Geometry: see drawing. Coordinates: mm, zero at the bounding-box minimum. Give positions to 0.01 mm unless a question says otherwise; leave off trailing zeros. Order: outer loops, then holes, each group sorted by start corner. A loop starts at its lowest first (then second) coordinate and runs counter-clockwise, first axis right, second up. Notation, with made-up numbers: M 42.5,-2 L 61.5,-2 A24 ccw 61.5,34 Z; hole C 73,39 d10. An arc over 180 degrees is marked long. Return JSON: item names as keys, results as strings.
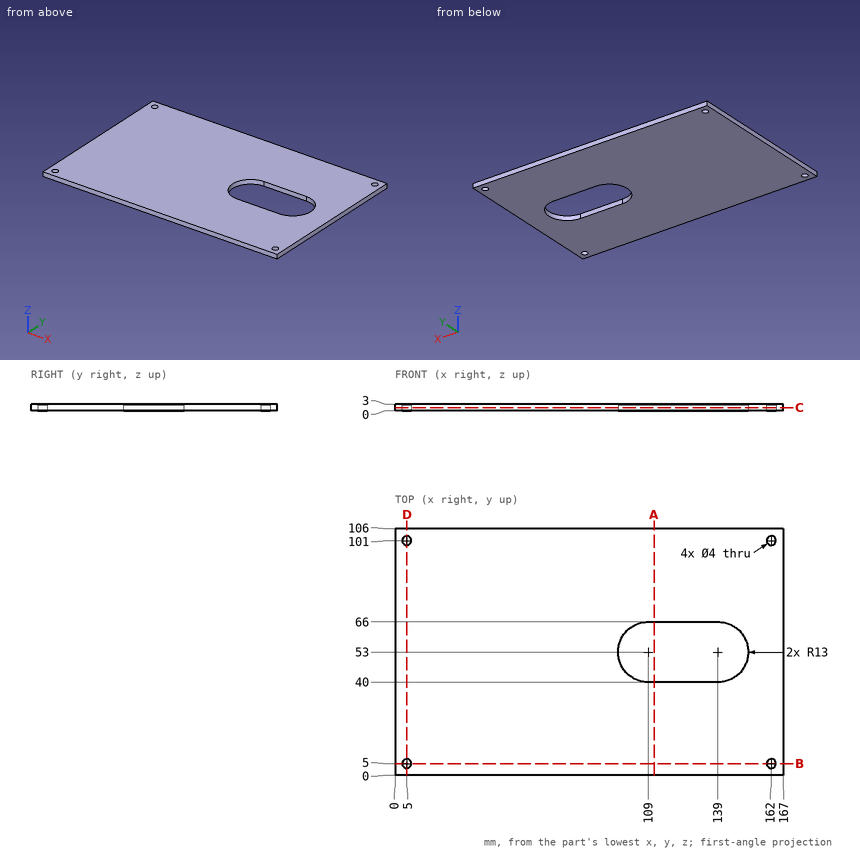
1. Section query D-D (x = 5). Return loops of the section in (y, z), then the cut area to 3 significant figures.
Evaluation:
{"outline": "M 0,0 L 3,0 L 3,3 L 0,3 Z; M 7,0 L 99,0 L 99,3 L 7,3 Z; M 103,0 L 106,0 L 106,3 L 103,3 Z", "area": "294 mm^2"}
2. Ray query, probe 1 along Y at (x, z) = (162, 1.75); probe 2 along X at (y, z) = (101, 1.2); probe 3 along Y at (x, z) = (119, 2.45). Return the intervals inside material, ascending.
Evaluation:
{"probe 1": "y = 0 to 3, 7 to 99, 103 to 106", "probe 2": "x = 0 to 3, 7 to 160, 164 to 167", "probe 3": "y = 0 to 40, 66 to 106"}
3. Section query C-C (z = 1.4). Return loops of the section in (x, y).
Evaluation:
{"outline": "M 0,0 L 167,0 L 167,106 L 0,106 Z; hole C 5,5 d4; hole C 5,101 d4; hole M 109,40 L 139,40 A13 ccw 139,66 L 109,66 A13 ccw Z; hole C 162,5 d4; hole C 162,101 d4"}
4. Section query A-A (x = 111.5). Return loops of the section in (y, z).
Evaluation:
{"outline": "M 0,0 L 40,0 L 40,3 L 0,3 Z; M 66,0 L 106,0 L 106,3 L 66,3 Z"}
5. Section query B-B (y = 5). Return loops of the section in (x, z).
Evaluation:
{"outline": "M 0,0 L 3,0 L 3,3 L 0,3 Z; M 7,0 L 160,0 L 160,3 L 7,3 Z; M 164,0 L 167,0 L 167,3 L 164,3 Z"}
6. First-contact query: pin 1 (3.5 mm diameter, centred on x = 5, y = 5, fed in from +Z). Flat tip, straight axial feed; report the tip coordinate or a pass-through.
Evaluation:
{"pin 1": "passes through"}
